from build123d import *

# Parameters (mm, degrees)
F0_R      = 15.5
F0_R_2    = 11
F1_DEPTH  = 25
F2_R      = 16.5
F2_R_2    = 11
F3_DEPTH  = 10
F5_R      = 15.5
F5_R_2    = 11
F6_DEPTH  = 25
F7_R      = 16.5
F7_R_2    = 11
F8_DEPTH  = 10
F9_R      = 11
F10_DEPTH = 200
F11_R     = 11
F12_DEPTH = 35


with BuildPart() as f1:
    # F0 (on Front) → F1 (new body)
    with BuildSketch(Plane.XZ):
        Circle(F0_R)
        Circle(F0_R_2, mode=Mode.SUBTRACT)
    extrude(amount=F1_DEPTH)

    # F2 (on face) → F3 (join)
    with BuildSketch(Plane.XZ.offset(25)):
        Circle(F2_R)
        Circle(F2_R_2, mode=Mode.SUBTRACT)
    extrude(amount=F3_DEPTH)

    # F4: F1 across plane


with BuildPart() as f1_1:
    add(f1.part)
    add(f1.part.mirror(Plane.XZ))

    # F5 (on Right) → F6 (join)
    with BuildSketch(Plane.YZ):
        Circle(F5_R)
        Circle(F5_R_2, mode=Mode.SUBTRACT)
    extrude(amount=F6_DEPTH)

    # F7 (on face) → F8 (join)
    with BuildSketch(Plane.YZ.offset(25)):
        Circle(F7_R)
        Circle(F7_R_2, mode=Mode.SUBTRACT)
    extrude(amount=F8_DEPTH)

    # F9 (on face) → F10 (cut)
    with BuildSketch(Plane.XZ.offset(35)):
        Circle(F9_R)
    extrude(amount=-F10_DEPTH, mode=Mode.SUBTRACT)

    # F11 (on face) → F12 (cut)
    with BuildSketch(Plane.YZ.offset(35)):
        Circle(F11_R)
    extrude(amount=-F12_DEPTH, mode=Mode.SUBTRACT)


solid = f1_1.part
Geometry: final body of the model. Coordinates: model frame, mm. A direction names the side the tool comes from. Coordinates: 2 decimals unless noted, no trailing zeros. Loops run counter-clockwise (first coordinate to the right, second up) from the corner with the lowest first, then second, coordinate; pieces in that order, holes last. Notation, with made-up numbers: (87.5, -24) - (125.5, -24) arc R19 cw to (125.5, -13) - close; hole circle Ø3 at (13, 77). An arc over 180 degrees is marked (long way). Put each result on its own line as item: value. Start each with the question number.
Q1. Cut plane D-D, the plane x = 20. Return loops of the section in (y, z).
Q2. Cut plane B-B, the plane x = 4.5. Return loops of the section in (y, z), and give its area (3 significant figures).
Q3. Cut plane C-C, the plane y = 0. Return loops of the section in (x, z), and give its area (3 significant figures).
Q4. Line query: line 1 (Y direction, x = 22.5, z = 0); line 2 (X direction, y = -24.5, z = 9). Output: solid intervals per line, ascending.
Q5. Pull-direction query (Y, two-part tool) for faces 4 (the cylindrical face through (29.93, 15.24, -6.32)), 5 (the cylindrical face through (15.24, -29.93, -6.32)), 6 (the flat face through (11, -35, -3)), 7 (the flat face through (5, 25, 15)); classes: released by +Y, released by -Y, zero draft, split by the parting line, or undercut.
Q6. Cut plane A-A, the plane z = 9. Return loops of the section in (x, y), and give its area (3 significant figures).
Q7. Set-up query: faces 1 (the flat face through (25, 5, 15)), 2 (the cylindrical face through (-11, 0, 0)), 3 (the cylindrical face through (15.24, 29.93, -6.32)). Return all of +Z, -Z, +X, -X, +Y, -Y with unobstructed straight access to the full face (end or side cutting, diameter ignored); none if empty.
Q8. Pin query (flat end, axial travel): pin 1 Ø6 at (y, z) = (4.5, -4.5) entering from +X; pin 2 Ø1.5 at (x, y) = (15, 18) entering from -Z; pin 3 Ø10 at (x, z) = (20, -12) entering from -Y; pin 4 Ø16.5 at (x, z) = (8, 3.5) entering from +Y. Return the tip coordinate at first contact, or that it passes through.
Filled sheet:
1. outline: circle Ø31 at (0, 0); hole circle Ø22 at (0, 0)
2. outline: (-35, -15.87) - (-25, -15.87) - (-25, -14.83) - (-4.5, -14.83) arc R15.5 ccw to (4.5, -14.83) - (25, -14.83) - (25, -15.87) - (35, -15.87) - (35, -10.04) - (4.5, -10.04) arc R11 cw to (-4.5, -10.04) - (-35, -10.04) - close; (-35, 10.04) - (-4.5, 10.04) arc R11 cw to (4.5, 10.04) - (35, 10.04) - (35, 15.87) - (25, 15.87) - (25, 14.83) - (4.5, 14.83) arc R15.5 ccw to (-4.5, 14.83) - (-25, 14.83) - (-25, 15.87) - (-35, 15.87) - close
2. area: 709 mm²
3. outline: (0, -15.5) - (25, -15.5) - (25, -16.5) - (35, -16.5) - (35, -11) - (0, -11) arc R11 cw to (0, 11) - (35, 11) - (35, 16.5) - (25, 16.5) - (25, 15.5) - (0, 15.5) arc R15.5 ccw to start
3. area: 522 mm²
4. line 1: -15.5 to -11, 11 to 15.5
4. line 2: -12.62 to -6.32, 6.32 to 12.62
5. face 4: split by the parting line
5. face 5: zero draft
5. face 6: released by -Y
5. face 7: undercut
6. outline: (-13.83, -35) - (-6.32, -35) - (-6.32, 35) - (-13.83, 35) - (-13.83, 25) - (-12.62, 25) - (-12.62, -25) - (-13.83, -25) - close; (6.32, -35) - (13.83, -35) - (13.83, -25) - (12.62, -25) - (12.62, -12.62) - (25, -12.62) - (25, -13.83) - (35, -13.83) - (35, -6.32) - (6.32, -6.32) - close; (6.32, 6.32) - (35, 6.32) - (35, 13.83) - (25, 13.83) - (25, 12.62) - (12.62, 12.62) - (12.62, 25) - (13.83, 25) - (13.83, 35) - (6.32, 35) - close
6. area: 1,160 mm²
7. face 1: none
7. face 2: +Y, -Y
7. face 3: +Y
8. pin 1: x = -8.05
8. pin 2: z = -6.1
8. pin 3: y = -13.83
8. pin 4: y = 35
